Answer from the drawing. Dimensions are ordinates in mm from the lowest x, y and z of the part. A direction names the side the tool comes from. Give positions to 0.01 mm unless a question says otherwise; leave off trailing zeros. Loops run counter-clockwise (first coordinate to the right, second up) from the corner with the lowest first, then second, coordinate; pieces in that order, holes last.
(1) Find section B-B, the plane y = 57.5. Write down the section's boundary in (x, z), then the cut area to 3 significant figures.
(2) Find section C-C, the plane x = 19.5. Write down the section's boundary in (y, z), then the cut area to 3 significant figures.
(3) Determine the mould class of the marked faces 3, 4 and 5 for opening direction X: pulls with the +X half, pulls with the -X half, needs draft (parallel to the pull), parting line crosses it, or undercut.
(4) Straight lines are drawn through the part: probe 1 along X at (y, z) = (9.5, 6); probe 2 along Y at (x, z) = (42, 7.75); probe 3 along Y at (x, z) = (52, 7). For each, find the intervals that lie inside material, in ascending order.
(5) Which of the six approach directions +Z, -Z, +X, -X, +Y, -Y give full straight-line access (tool end or side, diameter ignored) to the marked faces 1 and 2?
(6) Each of these flat-tipped pins is pushed along its axis until it touches: P1, Ø10, axis at x = 22, y = 14.5, coming from the +Z side; P2, Ø3.5, axis at x = 37, z = 8.5, coming from the +Y side; P3, Ø6, axis at x = 24, z = 9, coming from the -Y side. Where does it stop, or does it pass through?
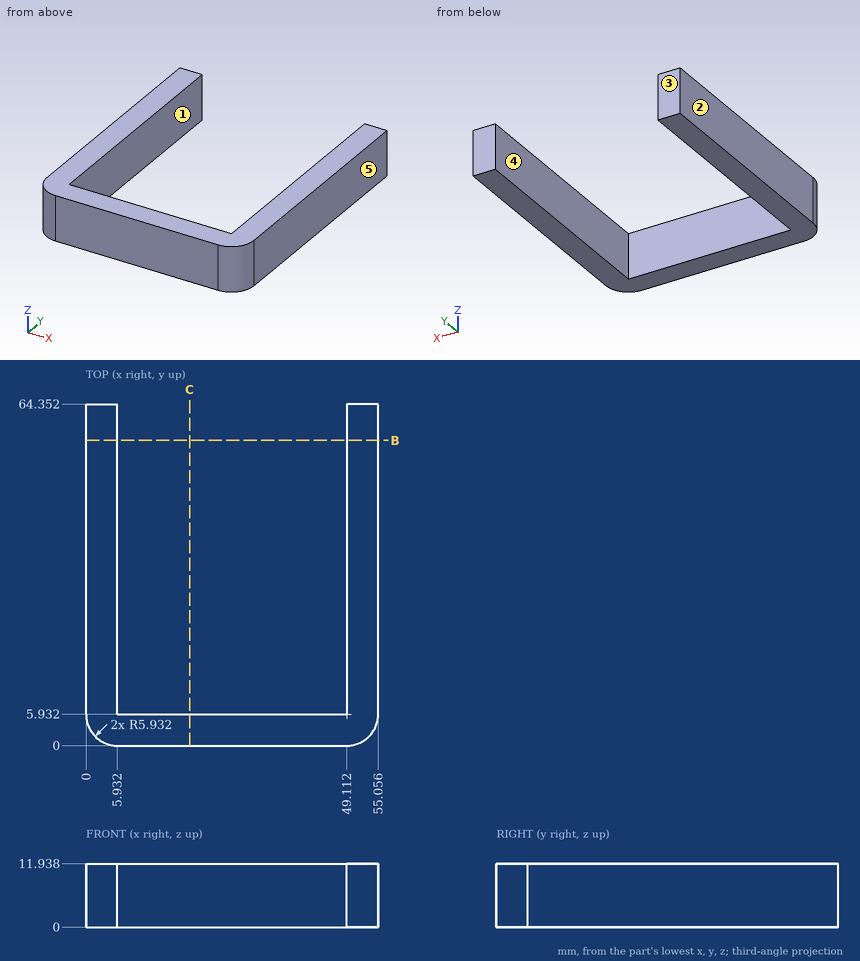
Entries:
1. outline: (0, 0) - (5.93, 0) - (5.93, 11.94) - (0, 11.94) - close; (49.11, 0) - (55.06, 0) - (55.06, 11.94) - (49.11, 11.94) - close
1. area: 142 mm2
2. outline: (0, 0) - (5.93, 0) - (5.93, 11.94) - (0, 11.94) - close
2. area: 70.8 mm2
3. face 3: needs draft
3. face 4: undercut
3. face 5: pulls with the +X half
4. probe 1: x = 0 to 5.93, 49.11 to 55.06
4. probe 2: y = 0 to 5.93
4. probe 3: y = 0.75 to 64.35
5. face 1: +Z, -Z, +Y
5. face 2: +Z, -Z, -X, +Y, -Y
6. P1: passes through
6. P2: stops at y = 5.93
6. P3: stops at y = 0
